Can you work these out from the model? Positions are in its coordinate system, mm. A direction names the side the tool comes from. Coordinates: 2 decimals unless noted, no trailing zeros. Loops run counter-clockwise (first coordinate to the right, second up) from the corner with the lowest first, then second, coordinate; pieces in that order, holes last. Notation, with made-up numbers: M 15,-37 L 38,-37 A19 ccw 38,-20 Z; hole C 30.5,-14 d4. An arc over 180 degrees is marked long. Answer as a JSON object with one key per item and string values. Group by question number.
Item 1: Suppose I cut it at B-B (x = 0). Write out the boundary of the cut face in (y, z).
Item 2: Which directions (+Z, -Z, +X, -X, +Y, -Y) give clear straight access to the entire face, cutting with the end or side of a thin tool? Please do faces 1 (the flat face through (6, 0, 2)), 2 (the flat face through (11.67, 24.35, 0.99)).
Item 3: I'm going to push flat-ended pins straight in: pin 1 Ø1.5 at (x, z) = (-1, 3) entering from -Y; pin 2 Ø3 at (x, z) = (6.5, 2) entering from +Y; pin 3 Ø0.6 at (x, z) = (-0.5, 1) entering from +Y. Where does each tip first touch, or does it pass through?
Item 4: Suppose I cut it at C-C (y = 7). Write out the boundary of the cut face in (x, z), then the cut area to 3 significant figures.
Item 5: If I drill on line 1 (Y direction, x = 0, z = 5); line 2 (Y direction, x = -22.5, z = 1.1); line 3 (Y direction, x = 13.5, z = 1.75), over which ranges is the centre line in solid material (lowest first)?
Item 6: Suppose I cut it at A-A (z = 4.3). Write out the boundary of the cut face in (x, y), then the cut area to 3 significant figures.
Item 7: Suppose I cut it at D-D (y = 13). Write out the boundary of the cut face in (x, z), then the cut area to 3 significant figures.
```python
from build123d import *

# Parameters (mm, degrees)
F0_R     = 30
F1_DEPTH = 6
F2_R     = 28.25
F2_R_2   = 5
F3_DEPTH = 4
F5_W     = 3.095944
F5_H     = 4
F6_DEPTH = 25
F8_DEPTH = 25


with BuildPart() as f1:
    # F0 (on Top) → F1 (new body)
    with BuildSketch(Plane.XY):
        Circle(F0_R)
        with BuildLine():
            ThreePointArc((2, 1.661325), (2.445404, 0.883176), (2.6, 0))
            ThreePointArc((2.6, 0), (2.445404, -0.883176), (2, -1.661325))
            ThreePointArc((2, -1.661325), (-2.6, 0), (2, 1.661325))
        make_face(mode=Mode.SUBTRACT)
        with BuildLine():
            ThreePointArc((2, -1.661325), (2.445404, -0.883176), (2.6, 0))
            ThreePointArc((2.6, 0), (2.445404, 0.883176), (2, 1.661325))
            Line((2, 1.661325), (2, -1.661325))
        make_face()
    extrude(amount=F1_DEPTH)

    # F2 (on face) → F3 (cut)
    with BuildSketch(Plane.XY.offset(6)):
        Circle(F2_R)
        Circle(F2_R_2, mode=Mode.SUBTRACT)
    extrude(amount=-F3_DEPTH, mode=Mode.SUBTRACT)

    # F5 (on offset) → F6 (cut)
    with BuildSketch(Plane.XZ.offset(25)):
        with Locations((0, 8)):
            Rectangle(F5_W, F5_H)
        with Locations((0, 4)):
            Rectangle(F5_W, F5_H)
    extrude(amount=F6_DEPTH, mode=Mode.SUBTRACT)

    # F7 (on face) → F8 (cut)
    with BuildSketch(Plane(origin=(0, 0, 0), x_dir=(1, 0, 0), z_dir=(0, 0, -1))):
        with BuildLine():
            ThreePointArc((-2.78543, 13.964289), (0, 12.078461), (2.78543, 13.964289))
            Line((2.78543, 13.964289), (6.354331, 22.886542))
            ThreePointArc((6.354331, 22.886542), (6.053103, 25.682601), (3.568901, 27.000714))
            Line((3.568901, 27.000714), (0, 27.000714))
            Line((0, 27.000714), (-3.568901, 27.000714))
            ThreePointArc((-3.568901, 27.000714), (-6.053103, 25.682601), (-6.354331, 22.886542))
            Line((-6.354331, 22.886542), (-2.78543, 13.964289))
        make_face()
        with BuildLine():
            ThreePointArc((21.85528, 9.30151), (23.853514, 11.280333), (23.335182, 14.044391))
            Line((23.335182, 14.044391), (21.110008, 16.83467))
            Line((21.110008, 16.83467), (18.884835, 19.624949))
            ThreePointArc((18.884835, 19.624949), (16.305418, 20.745346), (13.931559, 19.237542))
            Line((13.931559, 19.237542), (9.181034, 10.884329))
            ThreePointArc((9.181034, 10.884329), (9.443321, 7.530798), (12.654408, 6.528855))
            Line((12.654408, 6.528855), (21.85528, 9.30151))
        make_face()
        with BuildLine():
            ThreePointArc((20.898757, -11.28775), (23.691742, -11.616255), (25.529595, -9.487645))
            Line((25.529595, -9.487645), (26.32375, -6.008224))
            Line((26.32375, -6.008224), (27.117905, -2.528803))
            ThreePointArc((27.117905, -2.528803), (26.385626, 0.186423), (23.726701, 1.10228))
            Line((23.726701, 1.10228), (14.233992, -0.391753))
            ThreePointArc((14.233992, -0.391753), (11.775629, -2.687711), (12.994359, -5.82294))
            Line((12.994359, -5.82294), (20.898757, -11.28775))
        make_face()
        with BuildLine():
            ThreePointArc((4.205044, -23.377103), (5.689606, -25.765567), (8.499702, -25.875291))
            Line((8.499702, -25.875291), (11.715171, -24.326803))
            Line((11.715171, -24.326803), (14.93064, -22.778315))
            ThreePointArc((14.93064, -22.778315), (16.59692, -20.512881), (15.655153, -17.863021))
            Line((15.655153, -17.863021), (8.568464, -11.372837))
            ThreePointArc((8.568464, -11.372837), (5.240648, -10.882318), (3.549292, -13.789943))
            Line((3.549292, -13.789943), (4.205044, -23.377103))
        make_face()
        with BuildLine():
            ThreePointArc((-15.655153, -17.863021), (-16.59692, -20.512881), (-14.93064, -22.778315))
            Line((-14.93064, -22.778315), (-11.715171, -24.326803))
            Line((-11.715171, -24.326803), (-8.499702, -25.875291))
            ThreePointArc((-8.499702, -25.875291), (-5.689606, -25.765567), (-4.205044, -23.377103))
            Line((-4.205044, -23.377103), (-3.549292, -13.789943))
            ThreePointArc((-3.549292, -13.789943), (-5.240648, -10.882318), (-8.568464, -11.372837))
            Line((-8.568464, -11.372837), (-15.655153, -17.863021))
        make_face()
        with BuildLine():
            ThreePointArc((-23.726701, 1.10228), (-26.385626, 0.186423), (-27.117905, -2.528803))
            Line((-27.117905, -2.528803), (-26.32375, -6.008224))
            Line((-26.32375, -6.008224), (-25.529595, -9.487645))
            ThreePointArc((-25.529595, -9.487645), (-23.691742, -11.616255), (-20.898757, -11.28775))
            Line((-20.898757, -11.28775), (-12.994359, -5.82294))
            ThreePointArc((-12.994359, -5.82294), (-11.775629, -2.687711), (-14.233992, -0.391753))
            Line((-14.233992, -0.391753), (-23.726701, 1.10228))
        make_face()
        with BuildLine():
            ThreePointArc((-13.931559, 19.237542), (-16.305418, 20.745346), (-18.884835, 19.624949))
            Line((-18.884835, 19.624949), (-21.110008, 16.83467))
            Line((-21.110008, 16.83467), (-23.335182, 14.044391))
            ThreePointArc((-23.335182, 14.044391), (-23.853514, 11.280333), (-21.85528, 9.30151))
            Line((-21.85528, 9.30151), (-12.654408, 6.528855))
            ThreePointArc((-12.654408, 6.528855), (-9.443321, 7.530798), (-9.181034, 10.884329))
            Line((-9.181034, 10.884329), (-13.931559, 19.237542))
        make_face()
    extrude(amount=-F8_DEPTH, mode=Mode.SUBTRACT)


solid = f1.part
```
From the geometry:
{
 "1": {"outline": "M -30,0 L -27,0 L -27,2 L -30,2 Z; M -12.08,0 L -2.6,0 L -2.6,6 L -5,6 L -5,2 L -12.08,2 Z; M 2.6,0 L 30,0 L 30,6 L 28.25,6 L 28.25,2 L 5,2 L 5,6 L 2.6,6 Z"},
 "2": {"face 1": "+Z", "face 2": "+Z, -Z"},
 "3": {"pin 1": "y = -29.96", "pin 2": "y = 29.58", "pin 3": "y = 30"},
 "4": {"outline": "M -29.17,0 L -26.1,0 L -26.1,2 L -27.37,2 L -27.37,6 L -29.17,6 Z; M -14.7,0 L 14.7,0 L 14.7,2 L -14.7,2 Z; M 26.1,0 L 29.17,0 L 29.17,6 L 27.37,6 L 27.37,2 L 26.1,2 Z", "area": "85.5 mm2"},
 "5": {"line 1": "-5 to -2.6, 2.6 to 5, 28.25 to 30", "line 2": "-19.84 to -15.09, -9.58 to -0.91, 11.82 to 19.84", "line 3": "-26.79 to -18.48, -6.78 to 0.61, 6.17 to 15.89, 23.47 to 26.79"},
 "6": {"outline": "C 0,0 d10; M -1.55,-29.96 L -1.55,-28.21 A28.25 cw long 1.55,-28.21 L 1.55,-29.96 A30 ccw long Z; hole M 2,-1.66 L 2,1.66 A2.6 ccw long Z", "area": "373 mm2"},
 "7": {"outline": "M -27.04,0 L -10.35,0 L -10.35,2 L -25.08,2 L -25.08,6 L -27.04,6 Z; M -3.6,0 L 3.6,0 L 3.6,2 L -3.6,2 Z; M 10.35,0 L 27.04,0 L 27.04,6 L 25.08,6 L 25.08,2 L 10.35,2 Z", "area": "96.8 mm2"}
}
